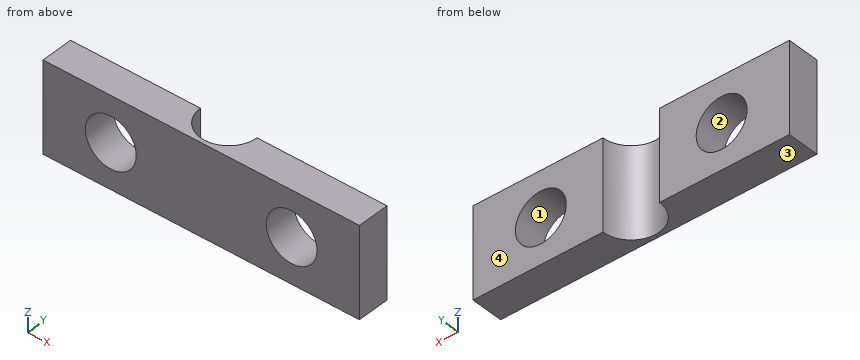
from build123d import *

# Parameters (mm, degrees)
BOSS_EXTRUDE1_DEPTH = 8
CUT_EXTRUDE1_REACH  = 31.26
SKETCH2_R           = 2.25


with BuildPart() as part:
    # Sketch1 → Boss-Extrude1 (new body)
    with BuildSketch(Plane.XY):
        with BuildLine():
            Line((0, 0), (-28, 0))
            Line((-28, 0), (-28, 2.85))
            Line((-28, 2.85), (-16.5, 2.85))
            ThreePointArc((-16.5, 2.85), (-14, 0.35), (-11.5, 2.85))
            Line((-11.5, 2.85), (0, 2.85))
            Line((0, 2.85), (0, 0))
        make_face()
    extrude(amount=BOSS_EXTRUDE1_DEPTH)

    # Sketch2 → Cut-Extrude1 (cut, up to next)
    with BuildSketch(Plane(origin=(0, 2.85, 0), x_dir=(1, 0, 0), z_dir=(0, 1, 0)), mode=Mode.PRIVATE) as cut_extrude1_sk1:
        with Locations(Location((-22, -4, 0), (0, 0, 270))):
            Circle(SKETCH2_R)
    cut_extrude1_tool1 = extrude(cut_extrude1_sk1.sketch, amount=-CUT_EXTRUDE1_REACH, mode=Mode.PRIVATE) & part.part
    # Sketch2 → Cut-Extrude1 (cut, up to next)
    with BuildSketch(Plane(origin=(0, 2.85, 0), x_dir=(1, 0, 0), z_dir=(0, 1, 0)), mode=Mode.PRIVATE) as cut_extrude1_sk2:
        with Locations(Location((-6, -4, 0), (0, 0, 270))):
            Circle(SKETCH2_R)
    cut_extrude1_tool2 = extrude(cut_extrude1_sk2.sketch, amount=-CUT_EXTRUDE1_REACH, mode=Mode.PRIVATE) & part.part
    add(cut_extrude1_tool1.solids().sort_by_distance((-22, 2.85, 4))[0], mode=Mode.SUBTRACT)
    add(cut_extrude1_tool2.solids().sort_by_distance((-6, 2.85, 4))[0], mode=Mode.SUBTRACT)


solid = part.part
Verification items for the finished model (mm, model axes). Face numbers are marked on the shaded views. Coordinates: 2 decimals unless noted, no trailing zeros. Order: outer loops, then holes, each group sorted by start corner. A loop starts at its lowest first (then second) coordinate and runs counter-clockwise, first axis right, second up. Notation, with made-up numbers: (56, -1.75) -> (63, -1.75) arc R24 cw to (63, 23.25) -> close; hole circle Ø2 at (76.25, -6). An arc over 180 degrees is marked (long way). Put each result on its own line as item: value. Start each with the question number.
1. Cross-section at C-C, the plane z = 4. Record the boundary of the cut face in (x, y), then the cut area to 3 significant figures.
2. Mould release check, pull along Z, two halves, no side actions. Record for the marked faces 1, 2, 3 and 4: released by +Z, released by -Z, zero draft, split by the parting line, or undercut.
3. Cross-section at B-B, the plane x = -22. Record the boundary of the cut face in (y, z).
4. Material ranges on L1, parallel to X at y = 2.4, z = 5.25; L2, parallel to X at y = 1.65, z = 4; L3, parallel to Z at x = -4.5, y = 1.4, recorded low to high. Write a range as [from, to].
5. Cross-section at D-D, the plane x = -14. Record the boundary of the cut face in (y, z).
6. Cross-section at A-A, the plane y = 1.15. Record the boundary of the cut face in (x, z).
Computed:
1. outline: (-28, 0) -> (-24.25, 0) -> (-24.25, 2.85) -> (-28, 2.85) -> close; (-19.75, 0) -> (-8.25, 0) -> (-8.25, 2.85) -> (-11.5, 2.85) arc R2.5 cw to (-16.5, 2.85) -> (-19.75, 2.85) -> close; (-3.75, 0) -> (0, 0) -> (0, 2.85) -> (-3.75, 2.85) -> close
1. area: 44.3 mm2
2. face 1: undercut
2. face 2: undercut
2. face 3: released by -Z
2. face 4: zero draft
3. outline: (0, 0) -> (2.85, 0) -> (2.85, 1.75) -> (0, 1.75) -> close; (0, 6.25) -> (2.85, 6.25) -> (2.85, 8) -> (0, 8) -> close
4. L1: [-28, -23.87], [-20.13, -16.46], [-11.54, -7.87], [-4.13, 0]
4. L2: [-28, -24.25], [-19.75, -16.19], [-11.81, -8.25], [-3.75, 0]
4. L3: [0, 2.32], [5.68, 8]
5. outline: (0, 0) -> (0.35, 0) -> (0.35, 8) -> (0, 8) -> close
6. outline: (-28, 0) -> (-15.83, 0) -> (-15.83, 8) -> (-28, 8) -> close; (-12.17, 0) -> (0, 0) -> (0, 8) -> (-12.17, 8) -> close; hole circle Ø4.5 at (-22, 4); hole circle Ø4.5 at (-6, 4)
